Geometry: final body of the model. Coordinates: model frame, mm. A direction names the side the tool comes from. Round coordinates to 2 decimals unless told otherwise and drop trailing zeros. Loops run counter-clockwise (first coordinate to the right, second up) from the corner with the lowest first, then second, coordinate; pieces in that order, holes last. Notation, with made-up numbers: M -28,-31 L 28,-31 A20 ccw 28,-10 Z; hole C -2.75,85 d5. An arc over 180 degrees is marked long. Answer as a JSON object with one key per item and string values.
```python
from build123d import *

# Parameters (mm, degrees)
SKETCH_W      = 165
SKETCH_H      = 105
PAD_DEPTH     = 2
SKETCH001_W   = 161
SKETCH001_H   = 101
SKETCH001_W_2 = 158
SKETCH001_H_2 = 98
PAD001_DEPTH  = 10.5
SKETCH002_W   = 2
SKETCH002_H   = 8
PAD002_DEPTH  = 16.5
SKETCH003_W   = 2
SKETCH003_H   = 9
PAD003_DEPTH  = 13.5


with BuildPart() as part:
    # Sketch → Pad (new body)
    with BuildSketch(Plane.XY):
        with Locations((82.5, 52.5)):
            Rectangle(SKETCH_W, SKETCH_H)
    extrude(amount=PAD_DEPTH)

    # Sketch001 → Pad001 (new body)
    with BuildSketch(Plane.XY.offset(2)):
        with Locations((82.5, 52.5)):
            Rectangle(SKETCH001_W, SKETCH001_H)
        with Locations((82.5, 52.5)):
            Rectangle(SKETCH001_W_2, SKETCH001_H_2, mode=Mode.SUBTRACT)
    extrude(amount=PAD001_DEPTH)

    # Sketch002 → Pad002 (new body)
    with BuildSketch(Plane.XY.offset(2)):
        with Locations((164, 84)):
            Rectangle(SKETCH002_W, SKETCH002_H)
    extrude(amount=PAD002_DEPTH)

    # Sketch003 → Pad003 (new body)
    with BuildSketch(Plane.XY.offset(2)):
        with Locations((164, 98)):
            Rectangle(SKETCH003_W, SKETCH003_H)
    extrude(amount=PAD003_DEPTH)


solid = part.part
```
1) Pull-direction query (Y, two-part tool) for faces 1 (the face through (165, 71.7, 1.7)), 2 (the face through (81, 2, 7)), 3 (the face through (161.5, 52, 7)); classes: +Y half, -Y half, draft (parallel to the pull), parting line (faces both ways), or undercut.
Geometry results:
{"face 1": "draft", "face 2": "-Y half", "face 3": "undercut"}
2) First-contact query: pin 1 (3 mm diameter, centred on x = 79.5, z = 8, fed in from -Y); pin 2 (5 mm diameter, centred on y = 48, z = 6.5, fed in from -X); pin 3 (8 mm diameter, centred on x = 27, y = 94, fed in from +Z). Flat tips, straight axial feed; report the tip coordinate or a pass-through.
Geometry results:
{"pin 1": "y = 2", "pin 2": "x = 2", "pin 3": "z = 2"}
3) Cut plane A-A on z = 7. Return the cut outline in (x, y).
Geometry results:
{"outline": "M 2,2 L 163,2 L 163,80 L 165,80 L 165,88 L 163,88 L 163,93.5 L 165,93.5 L 165,102.5 L 163,102.5 L 163,103 L 2,103 Z; hole M 3.5,3.5 L 161.5,3.5 L 161.5,101.5 L 3.5,101.5 Z"}
4) Set-up query: faces 4 (the face through (81, 103, 7)), 5 (the face through (163, 98, 14)), 6 (the face through (163, 40, 7)), 7 (the face through (81, 101.5, 7)). Return all of +Z, -Z, +X, -X, +Y, -Y with unobstructed straight access to the full face (end or side cutting, diameter ignored); none if empty.
Geometry results:
{"face 4": "+Z, +X, -X, +Y", "face 5": "+Z, -X, +Y, -Y", "face 6": "+Z, +X, -Y", "face 7": "+Z"}
5) Cut plane C-C on y = 76. Return the cut outline in (x, z), and give its area (4 significant figures).
Geometry results:
{"outline": "M 0,0 L 165,0 L 165,2 L 163,2 L 163,12.5 L 161.5,12.5 L 161.5,2 L 3.5,2 L 3.5,12.5 L 2,12.5 L 2,2 L 0,2 Z", "area": "361.5 mm2"}
6) Line query: probe 1 along Y at (x, z) = (93, 12.25); probe 2 along X at (y, z) = (13, 8.75); probe 3 along X at (y, z) = (82, 8). Output: solid intervals per line, ascending.
Geometry results:
{"probe 1": "2 to 3.5, 101.5 to 103", "probe 2": "2 to 3.5, 161.5 to 163", "probe 3": "2 to 3.5, 161.5 to 165"}
7) Cut plane B-B on x = 126. Return the cut outline in (y, z).
Geometry results:
{"outline": "M 0,0 L 105,0 L 105,2 L 103,2 L 103,12.5 L 101.5,12.5 L 101.5,2 L 3.5,2 L 3.5,12.5 L 2,12.5 L 2,2 L 0,2 Z"}
